Verification items for the finished model (mm, model axes). Face numbers are marked on the shaded views. A direction names the side the tool comes from. Coordinates: 2 decimals unless noted, no trailing zeros. Order: outer loops, then holes, each group sorted by start corner. A loop starts at its lowest first (then second) coordinate and runs counter-clockwise, first axis right, second up.
Q1. Depth check by flat-ended pin: P1, Ø1.5, axis at x = -1.5, z = 1.5, coming from the -Y side; P2, Ø1, axis at y = 7.5, z = 2, coming from the +X side; P3, Ø0.6, axis at x = 4, z = 2, coming from the +Y side. Enter the tip coordinate at first touch or a pass-through.
Q2. Cross-section at B-B, the plane x = 0. Record the boundary of the cut face in (y, z), and give its area (3 significant figures).
Q3. Thickness scan on line 1 (Y direction, x = 0.25, z = -0.5); line 2 (X direction, y = 3.25, z = 3.5); line 3 (X direction, y = -2.5, z = 1.75). Record the ranges inside material, lowest first.
Q4. Draft check along Y on the marked faces 1, 2 and 3. Enter one of: pulls with the +Y half, pulls with the -Y half, needs draft (parallel to the pull), parting line crosses it, or undercut.
Q5. Cross-section at C-C, the plane y = -4. Record the boundary of the cut face in (x, z).
Q6. Cross-section at A-A, the plane z = -0.25. Record the boundary of the cut face in (x, y), and give its area (3 significant figures).
Q7. Cross-section at D-D, the plane x = -9. Record the boundary of the cut face in (y, z), and give its area (3 significant figures).
Q8. Set-up check for the marked faces 4 and 5: record each of +Z, -Z, +X, -X, +Y, -Y from which the full face is reachable in a straight line by a thin tool's end or side.
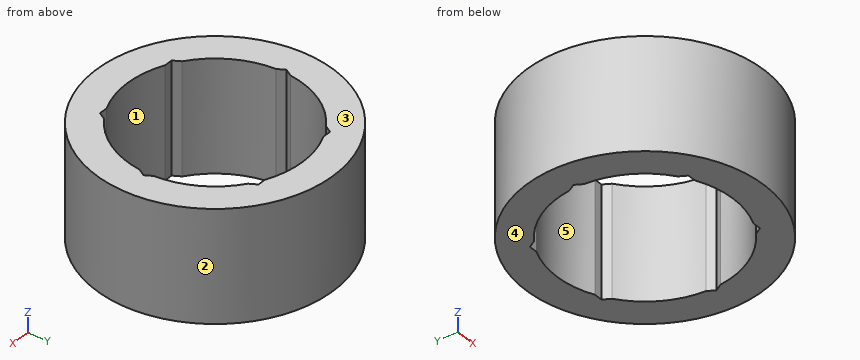
from build123d import *

# Parameters (mm, degrees)
SKETCH1_R           = 10.668
SKETCH1_R_2         = 7.8994
EXTRUDE_THIN1_DEPTH = 5
CUT_EXTRUDE3_DEPTH  = 11


with BuildPart() as part:
    # Sketch1 → Extrude-Thin1 (new body, symmetric)
    with BuildSketch(Plane.XY):
        Circle(SKETCH1_R)
        Circle(SKETCH1_R_2, mode=Mode.SUBTRACT)
    extrude(amount=EXTRUDE_THIN1_DEPTH, both=True)

    # Sketch3 → Cut-Extrude3 (cut, through all)
    with BuildSketch(Plane.XY.offset(5)):
        Polygon((4.124445986, 7.14375), (-4.124445986, 7.14375), (-8.248891971, 0), (-4.124445986, -7.14375), (4.124445986, -7.14375), (8.248891971, 0), align=None)
    extrude(amount=-CUT_EXTRUDE3_DEPTH, mode=Mode.SUBTRACT)


solid = part.part
Check values:
1. P1: stops at y = -10.64
1. P2: stops at x = 8.05
1. P3: stops at y = 10.01
2. outline: (-10.67, -5) - (-7.9, -5) - (-7.9, 5) - (-10.67, 5) - close; (7.9, -5) - (10.67, -5) - (10.67, 5) - (7.9, 5) - close
2. area: 55.4 mm2
3. line 1: y = -10.67 to -7.9, 7.9 to 10.67
3. line 2: x = -10.16 to -7.2, 7.2 to 10.16
3. line 3: x = -10.37 to -7.49, 7.49 to 10.37
4. face 1: undercut
4. face 2: parting line crosses it
4. face 3: needs draft
5. outline: (-9.89, -5) - (-6.81, -5) - (-6.81, 5) - (-9.89, 5) - close; (6.81, -5) - (9.89, -5) - (9.89, 5) - (6.81, 5) - close
6. outline: circle Ø21.34 at (0, 0); hole (-8.25, 0) - (-7.87, -0.65) arc R7.9 ccw to (-4.5, -6.49) - (-4.12, -7.14) - (-3.37, -7.14) arc R7.9 ccw to (3.37, -7.14) - (4.12, -7.14) - (4.5, -6.49) arc R7.9 ccw to (7.87, -0.65) - (8.25, 0) - (7.87, 0.65) arc R7.9 ccw to (4.5, 6.49) - (4.12, 7.14) - (3.37, 7.14) arc R7.9 ccw to (-3.37, 7.14) - (-4.12, 7.14) - (-4.5, 6.49) arc R7.9 ccw to (-7.87, 0.65) - close
6. area: 160 mm2
7. outline: (-5.73, -5) - (5.73, -5) - (5.73, 5) - (-5.73, 5) - close
7. area: 115 mm2
8. face 4: -Z, +X, -X, +Y, -Y
8. face 5: +Z, -Z
